Check sheet for the modelled part. Datum: model origin and axes. Units: mm. Round coordinates to 2 decimals unless told otherwise and drop trailing zeros. Order: outer loops, then holes, each group sorted by start corner. A loop starts at its lowest first (then second) coordinate and runs counter-clockwise, first axis right, second up. Notation, with made-up numbers: (-32, 15) -> (13, 15) arc R13 cw to (13, 36) -> close; hole circle Ø1 at (45.5, 23). An arc over 180 degrees is marked (long way). Answer as CSV lines item,"result". Start each with the question number.
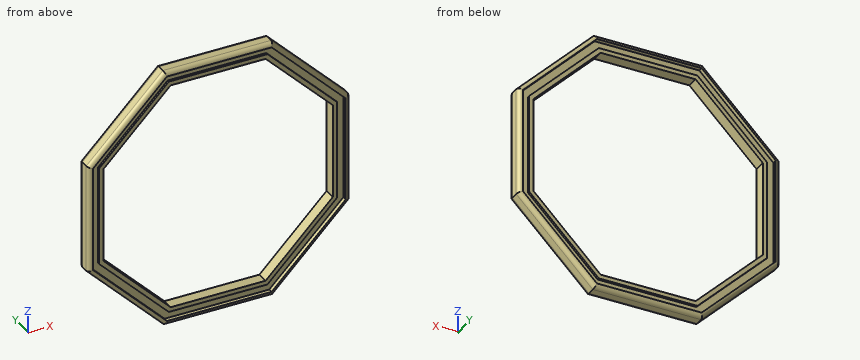
Autodesk Inventor part; units mm, degrees
ref_plane "작업 평면3" through (0, 2.2, 0) normal (0, -1, 0) x (1, 0, 0)
ref_plane "YZ Plane" through (0, 0, 0) normal (1, 0, 0) x (0, 1, 0)
ref_plane "XZ Plane" through (0, 0, 0) normal (0, 1, 0) x (-1, 0, 0)
sketch "스케치1" plane through (0, 0, 0) normal (0, 1, 0) x (-1, 0, 0)
  line L0 (-32.5919, 13.5) -> (-13.5, 32.5919)
  line L1 (-13.5, 32.5919) -> (13.5, 32.5919)
  line L2 (13.5, 32.5919) -> (32.5919, 13.5)
  line L3 (32.5919, 13.5) -> (32.5919, -13.5)
  line L4 (32.5919, -13.5) -> (13.5, -32.5919)
  line L5 (13.5, -32.5919) -> (-13.5, -32.5919)
  line L6 (-13.5, -32.5919) -> (-32.5919, -13.5)
  line L7 (-32.5919, -13.5) -> (-32.5919, 13.5)
  line L8 (35.7919, 14.8255) -> (35.7919, -14.8255)
  line L9 (35.7919, -14.8255) -> (14.8255, -35.7919)
  line L10 (14.8255, -35.7919) -> (-14.8255, -35.7919)
  line L11 (-14.8255, -35.7919) -> (-35.7919, -14.8255)
  line L12 (-35.7919, -14.8255) -> (-35.7919, 14.8255)
  line L13 (-35.7919, 14.8255) -> (-14.8255, 35.7919)
  line L14 (-14.8255, 35.7919) -> (14.8255, 35.7919)
  line L15 (14.8255, 35.7919) -> (35.7919, 14.8255)
  point P0 (0, 0)
  point P1 (0, 0)
  point P2 (0, 0)
  dimension "d0" = 27
  dimension "d1" = 3.2
extrude "돌출1" add sketch "스케치1" along normal blind 4.4 contours L0 L1 L2 L3 L4 L5 L6 L7 | L8 L9 L10 L11 L12 L13 L14 L15
sketch "스케치3" plane through (0, 0, 0) normal (0, -1, 0) x (1, 0, 0)
  line L0 (-13.5, 32.5919) -> (13.5, 32.5919)
  line L1 (13.5, 32.5919) -> (32.5919, 13.5)
  line L2 (32.5919, 13.5) -> (32.5919, -13.5)
  line L3 (32.5919, -13.5) -> (13.5, -32.5919)
  line L4 (13.5, -32.5919) -> (-13.5, -32.5919)
  line L5 (-13.5, -32.5919) -> (-32.5919, -13.5)
  line L6 (-32.5919, -13.5) -> (-32.5919, 13.5)
  line L7 (-32.5919, 13.5) -> (-13.5, 32.5919)
  line L8 (-14.3284, 34.5919) -> (14.3284, 34.5919)
  line L9 (14.3284, 34.5919) -> (34.5919, 14.3284)
  line L10 (34.5919, 14.3284) -> (34.5919, -14.3284)
  line L11 (34.5919, -14.3284) -> (14.3284, -34.5919)
  line L12 (14.3284, -34.5919) -> (-14.3284, -34.5919)
  line L13 (-14.3284, -34.5919) -> (-34.5919, -14.3284)
  line L14 (-34.5919, -14.3284) -> (-34.5919, 14.3284)
  line L15 (-34.5919, 14.3284) -> (-14.3284, 34.5919)
  point P0 (0, 0)
  point P1 (0, 0)
  point P2 (0, 0)
  point P3 (0, 0)
  dimension "d8" = 27
  dimension "d9" = 2
extrude "돌출3" cut sketch "스케치3" against normal blind 1.2
sketch "스케치14" plane through (0, 0, 0) normal (0, -1, 0) x (1, 0, 0)
  line L0 (32.5919, 13.5) -> (13.5, 32.5919)
  line L1 (13.5, 32.5919) -> (-13.5, 32.5919)
  line L2 (-13.5, 32.5919) -> (-32.5919, 13.5)
  line L3 (-32.5919, 13.5) -> (-32.5919, -13.5)
  line L4 (-32.5919, -13.5) -> (-13.5, -32.5919)
  line L5 (-13.5, -32.5919) -> (13.5, -32.5919)
  line L6 (13.5, -32.5919) -> (32.5919, -13.5)
  line L7 (32.5919, -13.5) -> (32.5919, 13.5)
  point P0 (0, 0)
extrude "돌출16" cut sketch "스케치14" against normal blind 0.6
sketch "스케치15" plane through (0, 0.6, 0) normal (0, -1, 0) x (1, 0, 0)
  line L0 (-13.0029, 31.3919) -> (13.0029, 31.3919)
  line L1 (13.0029, 31.3919) -> (31.3919, 13.0029)
  line L2 (31.3919, 13.0029) -> (31.3919, -13.0029)
  line L3 (31.3919, -13.0029) -> (13.0029, -31.3919)
  line L4 (13.0029, -31.3919) -> (-13.0029, -31.3919)
  line L5 (-13.0029, -31.3919) -> (-31.3919, -13.0029)
  line L6 (-31.3919, -13.0029) -> (-31.3919, 13.0029)
  line L7 (-31.3919, 13.0029) -> (-13.0029, 31.3919)
  line L8 (-13.5, 32.5919) -> (13.5, 32.5919)
  point P0 (0, 0)
  point P1 (0, 0)
  dimension "d140" = 1.2
extrude "돌출17" cut sketch "스케치15" against normal up to surface (3.8 mm away)
ref_plane "작업 평면3" through (0, 2.2, 0) normal (0, -1, 0) x (1, 0, 0)
mirror "미러6" about plane through (0, 2.2, 0) normal (0, -1, 0) of "돌출3", "돌출16"
fillet "모깎기2" radius 1.2 16 edges at (0, 0, 35.7919) (-25.3087, 0, 25.3087) (-35.7919, 0, 0) (-25.3087, 0, -25.3087) (0, 0, -35.7919) (25.3087, 0, -25.3087) (35.7919, 0, 0) (25.3087, 0, 25.3087) (-25.3087, 4.4, 25.3087) (-35.7919, 4.4, 0) (-25.3087, 4.4, -25.3087) (0, 4.4, -35.7919) (25.3087, 4.4, -25.3087) (35.7919, 4.4, 0) (25.3087, 4.4, 25.3087) (0, 4.4, 35.7919)
properties part number "OV-PAM_ring_2"
1) Depth check by flat-ended pin: pin 1 Ø1 at (y, z) = (0.5, 5) entering from -X; pin 2 Ø1 at (x, y) = (-5, 0.5) entering from -Z; pin 3 Ø1.5 at (x, y) = (-24, 3.5) entering from +Z. Enter the tip coordinate at first touch or a pass-through.
2) Section check A-A on y = 2.3. Record the cut outline in (x, z).
3) Material ranges on line 1 along X through (y, z) = (1.1, 0); line 2 along Z through (x, y) = (5, 1.35); line 3 along X through (y, z) = (0.8, -9.5), recorded low to high.
Solutions:
1,pin 1,"stops at x = -35.78"
1,pin 2,"stops at z = -35.78"
1,pin 3,"stops at z = 27.34"
2,outline,"(-35.79, -14.83) -> (-14.83, -35.79) -> (14.83, -35.79) -> (35.79, -14.83) -> (35.79, 14.83) -> (14.83, 35.79) -> (-14.83, 35.79) -> (-35.79, 14.83) -> close; hole (-31.39, -13) -> (-13, -31.39) -> (13, -31.39) -> (31.39, -13) -> (31.39, 13) -> (13, 31.39) -> (-13, 31.39) -> (-31.39, 13) -> close"
3,line 1,"x = -35.79 to -34.59, -32.59 to -31.39, 31.39 to 32.59, 34.59 to 35.79"
3,line 2,"z = -35.79 to -31.39, 31.39 to 35.79"
3,line 3,"x = -35.72 to -34.59, -32.59 to -31.39, 31.39 to 32.59, 34.59 to 35.72"
